Geometry check sheet. Reference: the model listing, model coordinates, mm. Round coordinates to 2 decimals unless told otherwise and drop trailing zeros. Loops run counter-clockwise (first coordinate to the right, second up) from the corner with the lowest first, then second, coordinate; pieces in that order, holes last. Notation, with made-up numbers: M 45.5,23.5 L 98.5,23.5 A14 ccw 98.5,31.5 Z; hole C 43.25,60 d3. An arc over 180 degrees is marked long. Write item = value, one per line.
from build123d import *

# Parameters (mm, degrees)
SKETCH1_R           = 4
BOSS_EXTRUDE1_DEPTH = 31.5
SKETCH2_W           = 6
SKETCH2_H           = 4.8
BOSS_EXTRUDE2_DEPTH = 21
SKETCH3_R           = 4
BOSS_EXTRUDE3_DEPTH = 8
SKETCH4_R           = 1.5
CUT_EXTRUDE1_DEPTH  = 61.968926512


with BuildPart() as part:
    # Sketch1 → Boss-Extrude1 (new body)
    with BuildSketch(Plane(origin=(0, 0, 0), x_dir=(0, 0, -1), z_dir=(1, 0, 0))):
        Circle(SKETCH1_R)
    boss_extrude1 = extrude(amount=BOSS_EXTRUDE1_DEPTH)

    # Sketch2 → Boss-Extrude2 (add)
    with BuildSketch(Plane(origin=(31.5, 0, 0), x_dir=(0, 0, -1), z_dir=(1, 0, 0))):
        Rectangle(SKETCH2_W, SKETCH2_H)
    boss_extrude2 = extrude(amount=BOSS_EXTRUDE2_DEPTH)

    # Sketch3 → Boss-Extrude3 (add)
    with BuildSketch(Plane(origin=(52.5, 0, 0), x_dir=(0, 0, -1), z_dir=(1, 0, 0))):
        Circle(SKETCH3_R)
    boss_extrude3 = extrude(amount=BOSS_EXTRUDE3_DEPTH)

    # Mirror1: Boss-Extrude1, Boss-Extrude2, Boss-Extrude3 across plane
    add(boss_extrude1.mirror(Plane(origin=(0, 0, 0), x_dir=(0, 0, 1), z_dir=(1, 0, 0))))
    add(boss_extrude2.mirror(Plane(origin=(0, 0, 0), x_dir=(0, 0, 1), z_dir=(1, 0, 0))))
    add(boss_extrude3.mirror(Plane(origin=(0, 0, 0), x_dir=(0, 0, 1), z_dir=(1, 0, 0))))

    # Sketch4 → Cut-Extrude1 (cut, through all)
    with BuildSketch(Plane(origin=(0, 2.4, 0), x_dir=(1, 0, 0), z_dir=(0, 1, 0))):
        with Locations(Location((-47, 0, 0), (0, 0, 270))):
            Circle(SKETCH4_R)
        with Locations(Location((-37, 0, 0), (0, 0, 270))):
            Circle(SKETCH4_R)
        with Locations(Location((47, 0, 0), (0, 0, 270))):
            Circle(SKETCH4_R)
        with Locations(Location((37, 0, 0), (0, 0, 270))):
            Circle(SKETCH4_R)
    extrude(amount=-CUT_EXTRUDE1_DEPTH, mode=Mode.SUBTRACT)


solid = part.part
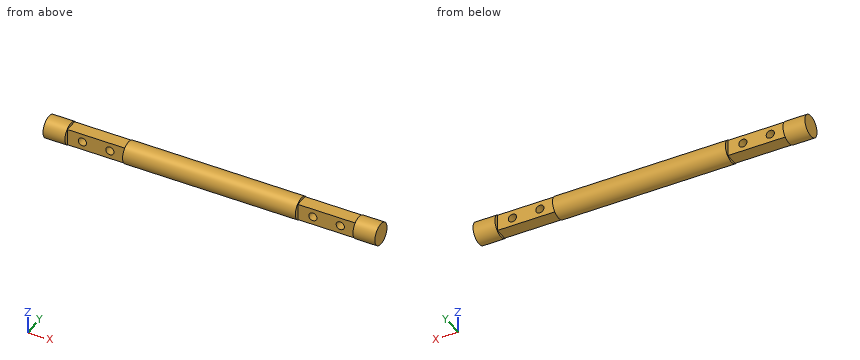
(1) Sectioned sample at A-A on x = -37. Record the cut outline in (y, z), then the cut area to 3 significant figures.
Result set:
outline = M -2.4,-3 L 2.4,-3 L 2.4,-1.5 L -2.4,-1.5 Z; M -2.4,1.5 L 2.4,1.5 L 2.4,3 L -2.4,3 Z
area = 14.4 mm2
(2) Sectioned sample at B-B on z = 0. State how many separate pieces and enclosed holes the cut face has, then the cut area to 3 significant figures.
Result set:
separate_pieces = 5
enclosed_holes = 0
area = 776 mm2
(3) Sectioned sample at C-C on y = -1. Record the cut outline in (x, z).
Result set:
outline = M -60.5,-3.87 L -52.5,-3.87 L -52.5,-3 L -31.5,-3 L -31.5,-3.87 L 31.5,-3.87 L 31.5,-3 L 52.5,-3 L 52.5,-3.87 L 60.5,-3.87 L 60.5,3.87 L 52.5,3.87 L 52.5,3 L 31.5,3 L 31.5,3.87 L -31.5,3.87 L -31.5,3 L -52.5,3 L -52.5,3.87 L -60.5,3.87 Z; hole C -47,0 d3; hole C -37,0 d3; hole C 37,0 d3; hole C 47,0 d3
(4) Sectioned sample at D-D on x = -0.5. Record the cut outline in (y, z), then the cut area to 3 significant figures.
Result set:
outline = C 0,0 d8
area = 50.3 mm2
(5) Material ranges on line 1 along X through (y, z) = (0, 0); line 2 along X through (y, z) = (2.75, -1.25); line 3 along X through (y, z) = (-2.25, -0.5), recorded low to high. Write a range as from..to.
Result set:
line_1 = -60.5..-48.5, -45.5..-38.5, -35.5..35.5, 38.5..45.5, 48.5..60.5
line_2 = -60.5..-52.5, -31.5..31.5, 52.5..60.5
line_3 = -60.5..-48.41, -45.59..-38.41, -35.59..35.59, 38.41..45.59, 48.41..60.5
(6) Depth check by flat-ended pin: pin 1 Ø2.5 at (x, y) = (37, 0) entering from -Z; pin 2 Ø3 at (x, z) = (-42, 0.5) entering from -Y; pin 3 Ø2.5 at (x, z) = (-47, 0) entering from -Y; pin 4 Ø2.5 at (x, y) = (37, 0) entering from +Z. Enter the tip coordinate at first touch or a pass-through.
Result set:
pin_1 = -3
pin_2 = -2.4
pin_3 = through
pin_4 = 3
